```python
from build123d import *

# Parameters (mm, degrees)
F2_R     = 10
F3_DEPTH = 77.978
F5_DEPTH = 40


# Not quite as in the source:
# - ends of sketch curves that miss each other by under 0.0002 mm in the source are joined


with BuildPart() as f1:
    # F0 (on Right) → F1 (revolve)
    with BuildSketch(Plane.YZ):
        Polygon((-29.7933634734, 31.385529514), (-37.9271134734, 31.385529514), (-37.9271134734, -53.704470486), (-29.7933634734, -53.704470486), (31.7266365266, -53.704470486), (39.8603865266, -53.704470486), (39.8603865266, 31.385529514), (31.7266365266, 31.385529514), (26.815313074, 17.891779514), (21.2579597972, 17.891779514), (16.3466364486, 31.385529514), (11.4353131, 17.891779514), (5.8779598232, 17.891779514), (0.9666364746, 31.385529514), (-3.944686874, 17.891779514), (-9.5020401508, 17.891779514), (-14.4133634994, 31.385529514), (-19.324686848, 17.891779514), (-24.8820401248, 17.891779514), align=None)
    revolve(axis=Axis((0, 0.9666365266, -53.704470486), (0, 1, 0)))

    # F2 (on face) → F3 (cut)
    with BuildSketch(Plane(origin=(0, 39.8603865266, 0), x_dir=(-1, 0, 0), z_dir=(0, 1, 0))):
        with Locations((0, -53.704470486)):
            Circle(F2_R)
    extrude(amount=-F3_DEPTH, mode=Mode.SUBTRACT)

    # F4 (on face) → F5 (cut)
    with BuildSketch(Plane.XZ.offset(37.9271134734)):
        with BuildLine():
            Line((2, -39.704470486), (0, -39.704470486))
            Line((0, -39.704470486), (-2, -39.704470486))
            Line((-2, -39.704470486), (-2, -43.9065115149))
            ThreePointArc((-2, -43.9065115149), (0, -43.704470486), (2, -43.9065115149))
            Line((2, -43.9065115149), (2, -39.704470486))
        make_face()
    extrude(amount=-F5_DEPTH, mode=Mode.SUBTRACT)


solid = f1.part
```
Here's how the part is built. I have some questions about the finished solid (model axes, mm). A direction names the side the tool comes from. Give positions to 0.01 mm unless a question says otherwise; leave off trailing zeros. Order: outer loops, then holes, each group sorted by start corner. A loop starts at its lowest first (then second) coordinate and runs counter-clockwise, first axis right, second up. Notation, with made-up numbers: (5, 58) -> (11, 58) arc R27 cw to (11, 89) -> close; hole circle Ø2 at (57.25, -13.75). An arc over 180 degrees is marked (long way). Use CSV: the item, a comma, the result in double quotes. Start each with the question number.
Item 1: Thinking about a two-plate mould opening in X: for faces 4 (the cylindrical face through (2.168, 1.511, -63.467)), 5 (the flat face through (1, 39.86, -71)), 6 (the conical face through (3.177, -19.086, -125.886)), which applies, pulls with the +X half, pulls with the -X half, needs draft (parallel to the pull), parting line crosses it, or undercut?
Item 2: On a 3-axis mill with a long thin cutter (end or side, diameter ignored), from which of +Z, -Z, +X, -X, +Y, -Y can I reach the whole of each face in a straight line? I mean faces 1 (the cylindrical face through (-32.59, -33.917, 24.897)), 2 (the flat face through (0, 2.073, -42)), 3 (the conical face through (21.76, 20.95, 15.39)). Say none if no direction works.
Item 3: Suppose I cut it at A-A (y = -16.5). List the corners of the cut face in (x, z) for me.
Item 4: I'm going to push flat-ended pins straight in: P1, Ø6, axis at y = 13.5, z = -16, coming from the +X side; P2, Ø8, axis at x = -62, y = 13, coming from the +Z side. Where does each tip first touch, or does it pass through?
Item 5: If I drill on probe 1 along Y at (x, z) = (12, 19.5); probe 2 along Y at (x, z) = (35, -124); probe 3 along Y at (x, z) = (-0.5, -43), over which ranges is the centre line in solid material (lowest first)? Write a range as [from, to].
Answer block:
1,face 4,"undercut"
1,face 5,"needs draft"
1,face 6,"parting line crosses it"
2,face 1,"+Y, -Y"
2,face 2,"-Y"
2,face 3,"none"
3,outline,"circle Ø158.71 at (0, -53.7); hole (-2, -43.91) arc R10 ccw (long way) to (2, -43.91) -> (2, -39.7) -> (-2, -39.7) -> close"
4,P1,"stops at x = 76.74"
4,P2,"stops at z = 6.82"
5,probe 1,"y = [-37.93, -25.82], [-18.38, -10.44], [-3, 4.94], [12.38, 20.32], [27.76, 39.86]"
5,probe 2,"y = [-37.93, -27.4], [-16.8, -12.02], [-1.42, 3.36], [13.96, 18.74], [29.34, 39.86]"
5,probe 3,"y = [2.07, 39.86]"
